Job drawing, mm, ordinate dimensions from the low corner. One solid piece. A direction names the side the tool comes from. Give positions to 0.01 mm unless a question says otherwise; leave off trailing zeros. Loops run counter-clockwise (first coordinate to the right, second up) from the corner with the lowest first, then second, coordinate; pieces in that order, holes last. Notation, with made-up numbers: (-10.5, 8.25) - (0.5, 8.25) arc R31 ccw to (0.5, 34.25) - close; hole circle Ø1 at (-15, -39.75). An arc over 180 degrees is marked (long way). Use a Markdown table: item, result.
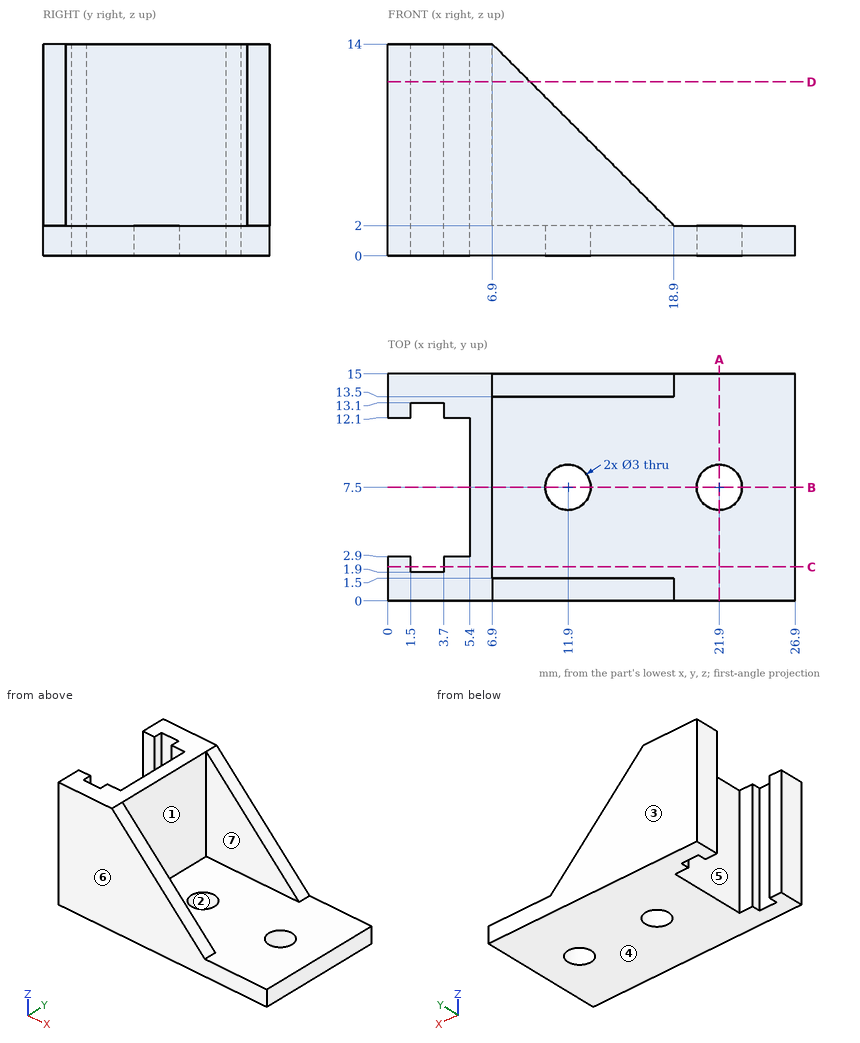
(1) Slice it at A-A, the plane x = 21.9. Write the cut outline in (y, z), plus the area to 3 significant figures.
Computed:
| item | result |
|---|---|
| outline | (0, 0) - (6, 0) - (6, 2) - (0, 2) - close; (9, 0) - (15, 0) - (15, 2) - (9, 2) - close |
| area | 24.0 mm² |
(2) 3-axis set-ups, long thin cutter, end or side, ignore diameter. For the marked faces 5, 6 and 7: which of +Z, -Z, +X, -X, +Y, -Y reach the whole face in a straight line?
Computed:
| item | result |
|---|---|
| face 5 | +Z, -Z, -X |
| face 6 | +Z, -Z, +X, -X, -Y |
| face 7 | +Z, +X |
(3) Mould opens along Y. For the marked faces 1, 2, 3 and 4 say: pulls with the +Y half, pulls with the -Y half, needs draft (parallel to the pull), parting line crosses it, or undercut.
Computed:
| item | result |
|---|---|
| face 1 | undercut |
| face 2 | undercut |
| face 3 | pulls with the +Y half |
| face 4 | needs draft |
(4) Drill centre lines: probe 1 along X at (y, z) = (7.5, 0.65); probe 2 along Y at (x, z) = (21.9, 1.3); probe 3 along X at (y, z) = (2.25, 3.25). Where is each one in solid material? Low to high. Write a range as [from, to].
Computed:
| item | result |
|---|---|
| probe 1 | [5.4, 10.4], [13.4, 20.4], [23.4, 26.9] |
| probe 2 | [0, 6], [9, 15] |
| probe 3 | [0, 1.5], [3.7, 6.9] |
(5) Slice it at D-D, the plane z = 11.5. Write the cut outline in (x, y), plus the area to 3 significant figures.
Computed:
| item | result |
|---|---|
| outline | (0, 0) - (9.4, 0) - (9.4, 1.5) - (6.9, 1.5) - (6.9, 13.5) - (9.4, 13.5) - (9.4, 15) - (0, 15) - (0, 12.1) - (1.5, 12.1) - (1.5, 13.1) - (3.7, 13.1) - (3.7, 12.1) - (5.4, 12.1) - (5.4, 2.9) - (3.7, 2.9) - (3.7, 1.9) - (1.5, 1.9) - (1.5, 2.9) - (0, 2.9) - close |
| area | 56.9 mm² |
(6) Slice it at C-C, the plane y = 2.25. Write the cut outline in (x, z), plus the area to 3 significant figures.
Computed:
| item | result |
|---|---|
| outline | (0, 0) - (1.5, 0) - (1.5, 14) - (0, 14) - close; (3.7, 0) - (26.9, 0) - (26.9, 2) - (6.9, 2) - (6.9, 14) - (3.7, 14) - close |
| area | 106 mm² |
(7) Pin check, flat tips, straight feed: P1, Ø0.8, axis at y = 2.5, z = 4.5, coming from the +X side; P2, Ø8, axis at x = 8, y = 11.5, coming from the -Z side; P3, Ø8, axis at x = 21, z = 6.5, coming from the +Y side; P4, Ø4, axis at x = 11.9, y = 7.5, coming from the +Z side. Stop position of each tip, or through.
Computed:
| item | result |
|---|---|
| P1 | x = 6.9 |
| P2 | z = 0 |
| P3 | through |
| P4 | z = 2 |
(8) Slice it at B-B, the plane y = 7.5. Write the cut outline in (x, z), plus the area to 3 significant figures.
Computed:
| item | result |
|---|---|
| outline | (5.4, 0) - (10.4, 0) - (10.4, 2) - (6.9, 2) - (6.9, 14) - (5.4, 14) - close; (13.4, 0) - (20.4, 0) - (20.4, 2) - (13.4, 2) - close; (23.4, 0) - (26.9, 0) - (26.9, 2) - (23.4, 2) - close |
| area | 49.0 mm² |
